Geometry check sheet. Reference: drawing and pictorial views, mm from the part's lowest x, y, z. Round coordinates to 2 decimals unless told otherwise and drop trailing zeros. Loops run counter-clockwise (first coordinate to the right, second up) from the corner with the lowest first, then second, coordinate; pieces in that order, holes last. Notation, with made-up numbers: M -30,32 L 15,32 A23 cw 15,64 Z; hole C 85,19 d2. An arc over 180 degrees is marked long. One line per question, with ' | ' between items. Start each with the question number.
(1) Section check A-A (x = 5). Record the boundary of the cut face in (y, z), and give its area (4 significant figures).
(2) Go/stop test with flat-tipped pins: P1, Ø1.5, axis at y = 3, z = 4, coming from the -X side; P2, Ø6, axis at x = 5, z = 4.5, coming from the -Y side; P3, Ø1.5, axis at y = 4, z = 7.5, coming from the +X side. Record where each tip stops, or that it passes through.
(3) Thickness scan on probe 1 along Z at (x, y) = (5, 3.3); probe 2 along Z at (x, y) = (5, 4.9); probe 3 along Z at (x, y) = (9, 3.35). Record the ranges inside material, lowest first. Write a range as [from, to].
(4) Section check B-B (z = 5). Record the boundary of the cut face in (x, y), and give its area (4 significant figures).
(5) Draft check along X on the marked faces 1, 2 and 3. Enter one of: +X half, -X half, draft (parallel to the pull), parting line (faces both ways), or undercut.
(6) Section check D-D (y = 0.9). Record the boundary of the cut face in (x, z), and give its area (3 significant figures).
(7) Section check C-C (y = 4.55). Record the boundary of the cut face in (x, z), and give its area (3 significant figures).
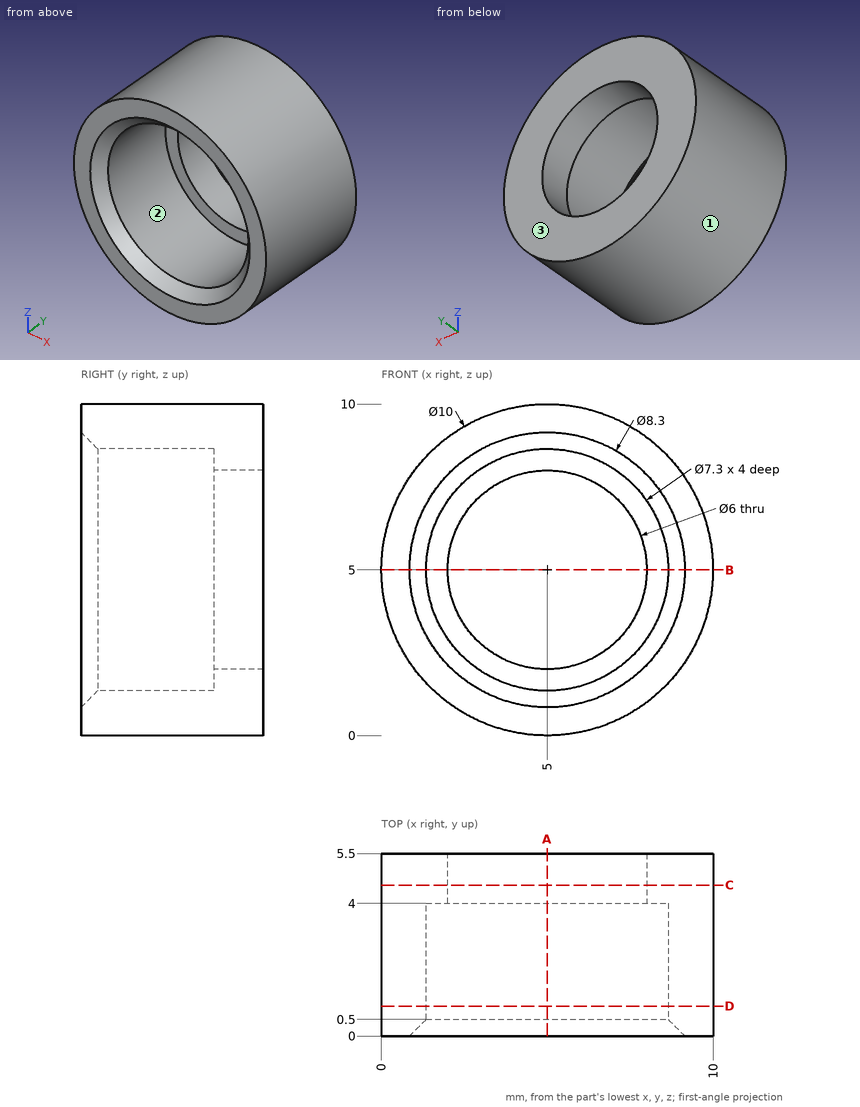
The answers:
1) outline: M 0,0 L 5.5,0 L 5.5,2 L 4,2 L 4,1.35 L 0.5,1.35 L 0,0.85 Z; M 0,9.15 L 0.5,8.65 L 4,8.65 L 4,8 L 5.5,8 L 5.5,10 L 0,10 Z | area: 16.55 mm²
2) P1: x = 0.01 | P2: y = 4 | P3: x = 9.68
3) probe 1: [0, 1.35], [8.65, 10] | probe 2: [0, 2], [8, 10] | probe 3: [2, 8]
4) outline: M 0,0 L 0.85,0 L 1.35,0.5 L 1.35,4 L 2,4 L 2,5.5 L 0,5.5 Z; M 8,4 L 8.65,4 L 8.65,0.5 L 9.15,0 L 10,0 L 10,5.5 L 8,5.5 Z | area: 16.55 mm²
5) face 1: parting line | face 2: undercut | face 3: draft
6) outline: C 5,5 d10; hole C 5,5 d7.3 | area: 36.7 mm²
7) outline: C 5,5 d10; hole C 5,5 d6 | area: 50.3 mm²
